Can you work these out from the model? Positions are in its coordinate system, mm. A direction names the side the tool comes from. Give positions to 0.01 mm unless a question says otherwise; leave off trailing zeros. Write each loop counter-clockwise with the first axis right and the second up, starting at its lowest first coordinate (ties: lowest second). Pieces come first, ordered by that corner, then holes. Notation, with made-up numbers: (85.5, 84) - (100.5, 84) arc R22 cw to (100.5, 102) - close; hole circle Ø6 at (50, 73). An arc over 180 degrees is marked (long way). Return JSON: item names as keys, results as strings. Group by question number.
from build123d import *

# Parameters (mm, degrees)
SKETCH1_R           = 1.55
SKETCH1_W           = 30
SKETCH1_H           = 25.5
BOSS_EXTRUDE1_DEPTH = 10
SKETCH2_W           = 59.5
SKETCH2_H           = 47.5
SKETCH2_W_2         = 53.5
SKETCH2_H_2         = 41.5
BOSS_EXTRUDE2_DEPTH = 4
CUT_EXTRUDE1_REACH  = 16
SKETCH3_R           = 1.5
FILLET2_R           = 1
SKETCH6_W           = 86.9
SKETCH6_H           = 10
BOSS_EXTRUDE3_DEPTH = 10
CUT_EXTRUDE2_REACH  = 61.15
SKETCH7_R           = 1.55


with BuildPart() as part:
    # Sketch1 → Boss-Extrude1 (new body)
    with BuildSketch(Plane(origin=(0, 0, 0), x_dir=(1, 0, 0), z_dir=(0, 1, 0))):
        Polygon((-43.45, 24.075), (43.45, 24.075), (43.45, -24.075), (43.45, -74.075), (-43.45, -74.075), (-43.45, -24.075), align=None)
        with Locations((-39.23, 19.985)):
            Circle(SKETCH1_R, mode=Mode.SUBTRACT)
        with Locations((-39.23, 8.835)):
            Circle(SKETCH1_R, mode=Mode.SUBTRACT)
        with Locations((-39.23, -8.835)):
            Circle(SKETCH1_R, mode=Mode.SUBTRACT)
        with Locations((-39.23, -19.985)):
            Circle(SKETCH1_R, mode=Mode.SUBTRACT)
        with Locations((39.23, -19.985)):
            Circle(SKETCH1_R, mode=Mode.SUBTRACT)
        with Locations((39.23, -8.835)):
            Circle(SKETCH1_R, mode=Mode.SUBTRACT)
        with Locations((39.23, 8.835)):
            Circle(SKETCH1_R, mode=Mode.SUBTRACT)
        with Locations((39.23, 19.985)):
            Circle(SKETCH1_R, mode=Mode.SUBTRACT)
        Rectangle(SKETCH1_W, SKETCH1_H, mode=Mode.SUBTRACT)
    extrude(amount=BOSS_EXTRUDE1_DEPTH)

    # Sketch2 → Boss-Extrude2 (add)
    with BuildSketch(Plane(origin=(0, 10, 0), x_dir=(1, 0, 0), z_dir=(0, 1, 0))):
        with Locations((0, -50)):
            Rectangle(SKETCH2_W, SKETCH2_H)
        with Locations((0, -50)):
            Rectangle(SKETCH2_W_2, SKETCH2_H_2, mode=Mode.SUBTRACT)
        Rectangle(SKETCH2_W, SKETCH2_H)
        Rectangle(SKETCH2_W_2, SKETCH2_H_2, mode=Mode.SUBTRACT)
    extrude(amount=BOSS_EXTRUDE2_DEPTH)

    # Sketch3 → Cut-Extrude1 (cut, up to next)
    with BuildSketch(Plane(origin=(0, 14, 0), x_dir=(1, 0, 0), z_dir=(0, 1, 0)), mode=Mode.PRIVATE) as cut_extrude1_sk1:
        with Locations((26.75, 20.75)):
            Circle(SKETCH3_R)
    cut_extrude1_tool1 = extrude(cut_extrude1_sk1.sketch, amount=-CUT_EXTRUDE1_REACH, mode=Mode.PRIVATE) & part.part
    add(cut_extrude1_tool1.solids().sort_by_distance((26.75, 14, -20.75))[0], mode=Mode.SUBTRACT)
    # Sketch3 → Cut-Extrude1 (cut, up to next)
    with BuildSketch(Plane(origin=(0, 14, 0), x_dir=(1, 0, 0), z_dir=(0, 1, 0)), mode=Mode.PRIVATE) as cut_extrude1_sk2:
        with Locations((26.75, -20.75)):
            Circle(SKETCH3_R)
    cut_extrude1_tool2 = extrude(cut_extrude1_sk2.sketch, amount=-CUT_EXTRUDE1_REACH, mode=Mode.PRIVATE) & part.part
    add(cut_extrude1_tool2.solids().sort_by_distance((26.75, 14, 20.75))[0], mode=Mode.SUBTRACT)
    # Sketch3 → Cut-Extrude1 (cut, up to next)
    with BuildSketch(Plane(origin=(0, 14, 0), x_dir=(1, 0, 0), z_dir=(0, 1, 0)), mode=Mode.PRIVATE) as cut_extrude1_sk3:
        with Locations((26.75, -29.25)):
            Circle(SKETCH3_R)
    cut_extrude1_tool3 = extrude(cut_extrude1_sk3.sketch, amount=-CUT_EXTRUDE1_REACH, mode=Mode.PRIVATE) & part.part
    add(cut_extrude1_tool3.solids().sort_by_distance((26.75, 14, 29.25))[0], mode=Mode.SUBTRACT)
    # Sketch3 → Cut-Extrude1 (cut, up to next)
    with BuildSketch(Plane(origin=(0, 14, 0), x_dir=(1, 0, 0), z_dir=(0, 1, 0)), mode=Mode.PRIVATE) as cut_extrude1_sk4:
        with Locations((26.75, -70.75)):
            Circle(SKETCH3_R)
    cut_extrude1_tool4 = extrude(cut_extrude1_sk4.sketch, amount=-CUT_EXTRUDE1_REACH, mode=Mode.PRIVATE) & part.part
    add(cut_extrude1_tool4.solids().sort_by_distance((26.75, 14, 70.75))[0], mode=Mode.SUBTRACT)

    # Fillet2
    fillet2_edges = [part.edges().sort_by_distance(p)[0] for p in [
        (-26.75, 14, 50),
        (-0.75, 14, 29.25),
        (26.75, 14, 50),
        (-0.75, 14, -20.75),
        (26.75, 14, 0),
        (-26.75, 14, 0),
        (-0.75, 14, 20.75),
        (-0.75, 14, 70.75),
    ]]
    fillet(fillet2_edges, radius=FILLET2_R)

    # Sketch6 → Boss-Extrude3 (add)
    with BuildSketch(Plane.XZ):
        with Locations((0, 30.075)):
            Rectangle(SKETCH6_W, SKETCH6_H)
    extrude(amount=BOSS_EXTRUDE3_DEPTH)

    # Sketch7 → Cut-Extrude2 (cut, up to next)
    with BuildSketch(Plane.XY.offset(35.075), mode=Mode.PRIVATE) as cut_extrude2_sk1:
        with Locations((-33.45, -5)):
            Circle(SKETCH7_R)
    cut_extrude2_tool1 = extrude(cut_extrude2_sk1.sketch, amount=-CUT_EXTRUDE2_REACH, mode=Mode.PRIVATE) & part.part
    add(cut_extrude2_tool1.solids().sort_by_distance((-33.45, -5, 35.075))[0], mode=Mode.SUBTRACT)
    # Sketch7 → Cut-Extrude2 (cut, up to next)
    with BuildSketch(Plane.XY.offset(35.075), mode=Mode.PRIVATE) as cut_extrude2_sk2:
        with Locations((33.45, -5)):
            Circle(SKETCH7_R)
    cut_extrude2_tool2 = extrude(cut_extrude2_sk2.sketch, amount=-CUT_EXTRUDE2_REACH, mode=Mode.PRIVATE) & part.part
    add(cut_extrude2_tool2.solids().sort_by_distance((33.45, -5, 35.075))[0], mode=Mode.SUBTRACT)


solid = part.part
1) I need wall thicknesses on line 1 along Z through (x, y) = (26.75, 8.75) (3 decimals); line 2 along Z through (x, y) = (-39.23, 3) (3 decimals); line 3 along Z through (x, y) = (-3, 9.5) (3 decimals). Which ranges of each line are inside material? Lowest first, please.
2) Imagine slicing it at D-D, the plane z = 42. Write out the boundary of the cut face in (x, y), and give its area (3 significant figures).
3) Imagine slicing it at B-B, the plane z = 0.5. Write out the boundary of the cut face in (x, y), and give its area (3 significant figures).
4) On a 3-axis mill with a long thin cutter (end or side, diameter ignored), from which of +Z, -Z, +X, -X, +Y, -Y can I reach the whole of each face in a straight line? I mean faces 4 (the face through (0, 5, -12.75)), 5 (the face through (0, 12, 26.25)), 6 (the face through (-1, -5, 35.075)). Say none if no direction works.
5) Imagine slicing it at A-A, the plane x = -39.23. Write out the boundary of the cut face in (y, z) (3 decimals), and give its area (4 significant figures).
6) Will these pins go through, and if not, where does the flat tip stop? pin 1 Ø5 at (x, z) = (11.5, 19) entering from -Y; pin 2 Ø3.5 at (x, z) = (-39.23, 8.835) entering from +Y; pin 3 Ø0.9 at (y, z) = (12, -2.5) entering from -X.
7) We'd pull the mould along X, two halves only. Please class faces 1 (the face through (-29.75, 12, 50)), 2 (the face through (0, 12, 73.75)), 3 (the face through (27.556, 7.098, 27.985)): pulls with the +X half, pulls with the -X half, needs draft (parallel to the pull), parting line crosses it, or undercut.
Resolved:
{
 "1": {"line 1": "-24.075 to -22.25, -19.25 to 19.25, 22.25 to 27.75, 30.75 to 69.25, 72.25 to 74.075", "line 2": "-24.075 to -21.535, -18.435 to -10.385, -7.285 to 7.285, 10.385 to 18.435, 21.535 to 74.075", "line 3": "-24.075 to -12.75, 12.75 to 74.075"},
 "2": {"outline": "(-43.45, 0) - (43.45, 0) - (43.45, 10) - (29.75, 10) - (29.75, 14) - (27.75, 14) arc R1 ccw to (26.75, 13) - (26.75, 10) - (-26.75, 10) - (-26.75, 13) arc R1 ccw to (-27.75, 14) - (-29.75, 14) - (-29.75, 10) - (-43.45, 10) - close", "area": "893 mm^2"},
 "3": {"outline": "(-43.45, 0) - (-15, 0) - (-15, 10) - (-26.75, 10) - (-26.75, 13) arc R1 ccw to (-27.75, 14) - (-29.75, 14) - (-29.75, 10) - (-43.45, 10) - close; (15, 0) - (43.45, 0) - (43.45, 10) - (29.75, 10) - (29.75, 14) - (27.75, 14) arc R1 ccw to (26.75, 13) - (26.75, 10) - (15, 10) - close", "area": "593 mm^2"},
 "4": {"face 4": "+Y, -Y", "face 5": "+X, -X, +Y", "face 6": "+Z, +X, -X, -Y"},
 "5": {"outline": "(-10, 25.075) - (0, 25.075) - (0, 21.535) - (10, 21.535) - (10, 74.075) - (0, 74.075) - (0, 35.075) - (-10, 35.075) - close; (0, -24.075) - (10, -24.075) - (10, -21.535) - (0, -21.535) - close; (0, -18.435) - (10, -18.435) - (10, -10.385) - (0, -10.385) - close; (0, -7.285) - (10, -7.285) - (10, 7.285) - (0, 7.285) - close; (0, 10.385) - (10, 10.385) - (10, 18.435) - (0, 18.435) - close", "area": "957.5 mm^2"},
 "6": {"pin 1": "y = 0", "pin 2": "y = 10", "pin 3": "x = -29.75"},
 "7": {"face 1": "pulls with the -X half", "face 2": "needs draft", "face 3": "undercut"}
}
